from build123d import *

# Parameters (mm, degrees)
SKICA3_R                      = 9
ODEBRAT_VYSUNUT_M1_DEPTH      = 25.75
ODEBRAT_VYSUNUT_M1_DEPTH_BACK = 25.75
ODEBRAT_VYSUNUT_M2_DEPTH      = 40
ZAOBLIT1_R                    = 2


with BuildPart() as part:
    # Skica2 → Rotovat1 (revolve)
    with BuildSketch(Plane.XY):
        Polygon((0, 0), (24.75, 0), (24.75, 47.5), (24, 47.5), (24, 48.5), (24.75, 48.5), (24.75, 50), (24, 50), (24, 51), (24.75, 51), (24.75, 52), (24, 52), (24, 53), (24.75, 53), (24.75, 55), (0, 55), align=None)
    revolve(axis=Axis((0, 49.551771463, 0), (0, -1, 0)))

    # Skica3 → Odebrat vysunutím1 (cut, two sides)
    with BuildSketch(Plane.XY) as odebrat_vysunut_m1_sk:
        with Locations((0, 15)):
            Circle(SKICA3_R)
    extrude(amount=ODEBRAT_VYSUNUT_M1_DEPTH, mode=Mode.SUBTRACT)
    extrude(odebrat_vysunut_m1_sk.sketch, amount=-ODEBRAT_VYSUNUT_M1_DEPTH_BACK, mode=Mode.SUBTRACT)

    # Skica4 → Odebrat vysunutím2 (cut)
    with BuildSketch(Plane.XZ):
        with BuildLine():
            Line((-13, 21.060923532), (13, 21.060923532))
            ThreePointArc((13, 21.060923532), (0, 24.75), (-13, 21.060923532))
        make_face()
        with BuildLine():
            ThreePointArc((15.686379442, 12), (19.75, 0), (15.686379442, -12))
            Line((15.686379442, -12), (-15.686379442, -12))
            ThreePointArc((-15.686379442, -12), (-19.75, 0), (-15.686379442, 12))
            Line((-15.686379442, 12), (15.686379442, 12))
        make_face()
        with BuildLine():
            Line((13, -21.060923532), (-13, -21.060923532))
            ThreePointArc((-13, -21.060923532), (0, -24.75), (13, -21.060923532))
        make_face()
    extrude(amount=-ODEBRAT_VYSUNUT_M2_DEPTH, mode=Mode.SUBTRACT)

    # Zaoblit1
    zaoblit1_edges = [part.edges().sort_by_distance(p)[0] for p in [
        (0, 40, 21.060923532),
        (0, 40, -12),
        (0, 40, 12),
        (19.75, 40, 0),
        (-19.75, 40, 0),
        (0, 40, -21.060923532),
    ]]
    fillet(zaoblit1_edges, radius=ZAOBLIT1_R)


solid = part.part
Work out the finished part from the listing and answer in its coordinate system (mm). A direction names the side the tool comes from. Round coordinates to 2 decimals unless told otherwise and drop trailing zeros. Loops run counter-clockwise (first coordinate to the right, second up) from the corner with the lowest first, then second, coordinate; pieces in that order, holes last. Notation, with made-up numbers: (61.5, 85.25) - (90.5, 85.25) arc R16 cw to (90.5, 91.25) - close; hole circle Ø7 at (52, 37). An arc over 180 degrees is marked (long way). One line per item, written item: value.
Q1. Find section D-D on x = 0. State how many separate pieces and enclosed holes the cut face has, and give its area (3 significant figures).
Check values:
separate pieces: 3
enclosed holes: 0
area: 1,140 mm2
Q2. The mould has two halves that part along Z. Classify faces 6 (the cylindrical face through (13.305, 24.082, 20.869)), 7 (the flat face through (0, 27, 12)), 8 (the flat face through (0, 0, -14)), 9 (the cylindrical face through (-19.75, 18.73, -0.18)): +Z half, -Z half, draft (parallel to the pull), parting line (faces both ways), or undercut.
Check values:
face 6: parting line
face 7: undercut
face 8: draft
face 9: undercut
Q3. Each of these flat-tipped pins is pushed along its axis until it touches: pin 1 Ø3 at (x, y) = (18.5, 36) entering from -Z; pin 2 Ø12 at (x, y) = (-12.5, 10.5) entering from -Z; pin 3 Ø1.9 at (x, z) = (4, -23.5) entering from -Y. Where does it stop, or does it pass through?
Check values:
pin 1: z = -17.99
pin 2: z = -21.06
pin 3: y = 39.93
Q4. Straight lines are drawn through the part: probe 1 along Z at (x, y) = (-12.5, 33); probe 2 along Y at (x, z) = (0, 15.5); probe 3 along Y at (x, z) = (12.5, -0.5). For each, find the intervals that lie inside material, in ascending order.
Check values:
probe 1: -21.06 to -12, 12 to 21.06
probe 2: 0 to 6, 24 to 55
probe 3: 40 to 55
Q5. Find section A-A on y = 15. Give the vertices of the cut face in (x, z), and give its area (3 significant figures).
Check values:
outline: (-15.69, -12) arc R19.75 cw to (-15.69, 12) - (-9, 12) - (-9, 21.06) - (-13, 21.06) arc R24.75 ccw to (-13, -21.06) - (-9, -21.06) - (-9, -12) - close; (9, -21.06) - (13, -21.06) arc R24.75 ccw to (13, 21.06) - (9, 21.06) - (9, 12) - (15.69, 12) arc R19.75 cw to (15.69, -12) - (9, -12) - close
area: 582 mm2
Q6. For faces 1 (the cylindrical face through (-1.172, 23.923, 16.467)), 2 (the flat face through (0, 40, 0)), 3 (the cylindrical face through (-23.977, 52.507, 1.055)), 4 (the flat face through (6, 23, -21.061)), 5 (the flat face through (0, 40, 24)), determine the directions among +Z, -Z, +X, -X, +Y, -Y from which every point of the face is accessible in a straight line to the end or side of a thin tool.
Check values:
face 1: +Z, -Z
face 2: -Y
face 3: none
face 4: -Z, +X, -X, -Y
face 5: +Z, +X, -X, -Y
Q7. Find section C-C on y = 35. Give the vertices of the cut face in (x, z), and give its area (3 significant figures).
Check values:
outline: (-13, -21.06) - (13, -21.06) arc R24.75 ccw to (13, 21.06) - (-13, 21.06) arc R24.75 ccw to start; hole (-15.69, -12) - (15.69, -12) arc R19.75 ccw to (15.69, 12) - (-15.69, 12) arc R19.75 ccw to start
area: 909 mm2
